Source: CAD feature listing. Evaluate the final solid. Frame: model axes, mm. Face numbers are marked on the shaded views. Coordinates: 2 decimals unless noted, no trailing zeros. Write each loop counter-clockwise with the first axis right and the second up, starting at its lowest first coordinate (ties: lowest second). Pieces come first, ordered by that corner, then holes. Notation, with made-up numbers: (-2, 81) -> (36, 81) arc R23 ccw to (36, 95) -> close; hole circle Ø1 at (5, 52.5). An arc over 180 degrees is marked (long way). Write item = value, one per line.
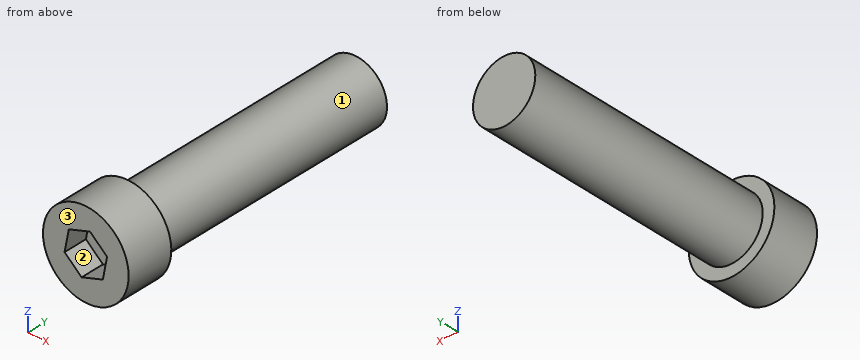
from build123d import *

# Parameters (mm, degrees)
SKETCH_1_R          = 2.75
EXTRUDE_1_DEPTH     = 3
SKETCH_2_R          = 2
EXTRUDE_2_DEPTH     = 16
CUT_EXTRUDE_1_DEPTH = 1.5


with BuildPart() as part:
    # 草图1 → 凸台-拉伸1 (new body)
    with BuildSketch(Plane(origin=(0, 0, 0), x_dir=(1, 0, 0), z_dir=(0, 1, 0))):
        with Locations(Location((0, 0, 0), (0, 0, 270))):
            Circle(SKETCH_1_R)
    extrude(amount=EXTRUDE_1_DEPTH)

    # 草图2 → 凸台-拉伸2 (add)
    with BuildSketch(Plane(origin=(0, 3, 0), x_dir=(1, 0, 0), z_dir=(0, 1, 0))):
        with Locations(Location((0, 0, 0), (0, 0, 270))):
            Circle(SKETCH_2_R)
    extrude(amount=EXTRUDE_2_DEPTH)

    # 草图3 → 切除-拉伸1 (cut)
    with BuildSketch(Plane.XZ):
        Polygon((1.091681609, -0.944226984), (1.36356536, 0.473310514), (0.271883751, 1.417537498), (-1.091681609, 0.944226984), (-1.36356536, -0.473310514), (-0.271883751, -1.417537498), align=None)
    extrude(amount=-CUT_EXTRUDE_1_DEPTH, mode=Mode.SUBTRACT)


solid = part.part
1) Cut plane C-C, the plane x = -0.8. Output: boundary loops of the cut face in (y, z), and give its area (3 significant figures).
Answer block:
outline = (0, -2.63) -> (3, -2.63) -> (3, -1.83) -> (19, -1.83) -> (19, 1.83) -> (3, 1.83) -> (3, 2.63) -> (0, 2.63) -> (0, 1.05) -> (1.5, 1.05) -> (1.5, -0.96) -> (0, -0.96) -> close
area = 71.4 mm2
2) Material intervals for probe 1 along Y at (x, z) = (1.45, 2.2); probe 2 along X at (y, z) = (16, -0.1); probe 3 along Y at (x, z) = (0.7, -0.15), sorted ascending. Write a range as [from, to].
Answer block:
probe_1 = [0, 3]
probe_2 = [-2, 2]
probe_3 = [1.5, 19]
3) Cut plane A-A, the plane y = 5. Output: boundary loops of the cut face in (x, z).
Answer block:
outline = circle Ø4 at (0, 0)
4) First-contact query: pin 1 Ø2 at (y, z) = (14.5, -0.5) entering from +X. Flat tip, straight axial feed; report the tip coordinate or a pass-through.
Answer block:
pin_1 = 2
5) Cut plane D-D, the plane z = -1.8. Output: boundary loops of the cut face in (x, y).
Answer block:
outline = (-2.08, 0) -> (2.08, 0) -> (2.08, 3) -> (0.87, 3) -> (0.87, 19) -> (-0.87, 19) -> (-0.87, 3) -> (-2.08, 3) -> close
6) Cut plane B-B, the plane z = 1.25. Output: boundary loops of the cut face in (x, y).
Answer block:
outline = (-2.45, 0) -> (-0.21, 0) -> (-0.21, 1.5) -> (0.47, 1.5) -> (0.47, 0) -> (2.45, 0) -> (2.45, 3) -> (1.56, 3) -> (1.56, 19) -> (-1.56, 19) -> (-1.56, 3) -> (-2.45, 3) -> close
7) Pull-direction query (Z, two-part tool) for the marked faces 1, 2 and 3; classes: +Z half, -Z half, draft (parallel to the pull), parting line (faces both ways), or undercut.
Answer block:
face_1 = parting line
face_2 = undercut
face_3 = draft
